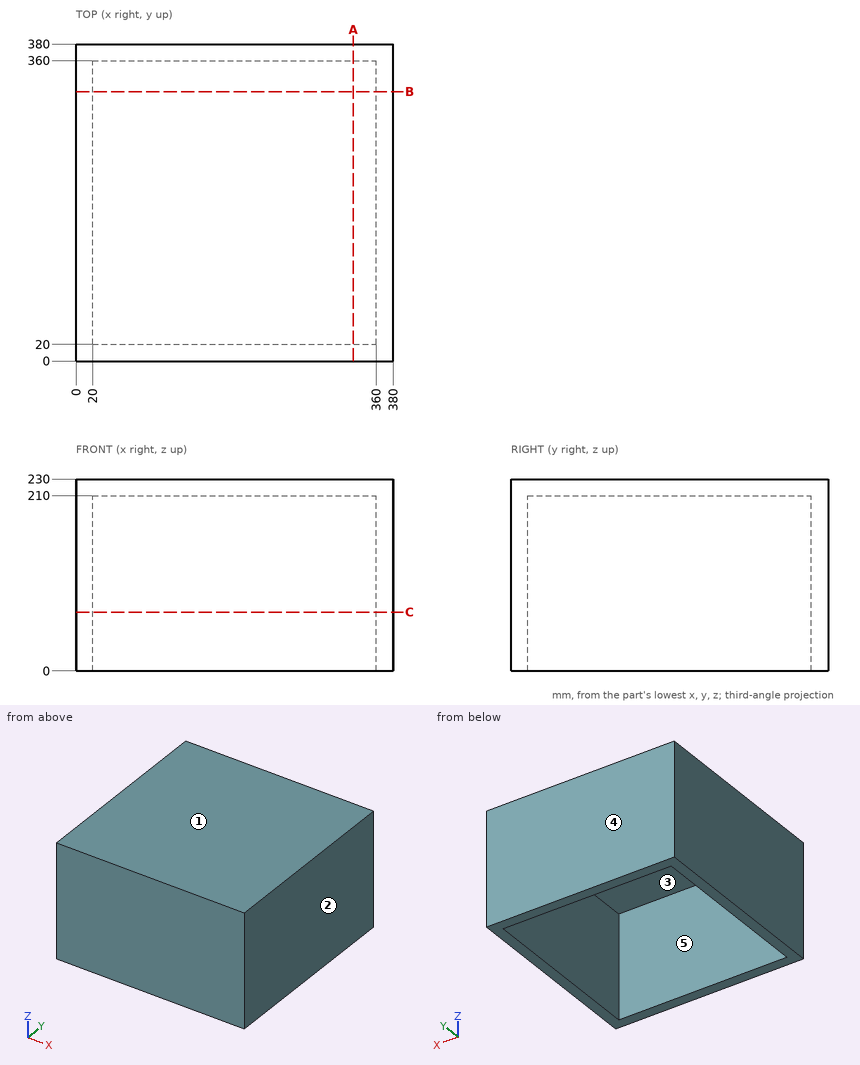
Design review of the part shown in the three views and the two pictorial views. Dimensions are in mm from the part's minimum x, y and z. A direction names the side the tool comes from. Round coordinates to 2 decimals unless told otherwise and drop trailing zeros. Loops run counter-clockwise (first coordinate to the right, second up) from the corner with the lowest first, then second, coordinate; pieces in that order, holes last. Notation, with made-up numbers: (20.5, 33) -> (71.5, 33) arc R24 ccw to (71.5, 52) -> close; hole circle Ø11 at (76.25, 49.25). An arc over 180 degrees is marked (long way). Return JSON: item names as keys, results as strings.
(1) For line 1 (X direction, y = 190, z = 71); line 2 (Z direction, x = 199.5, y = 124), list the stretches that pass through material, from the lowest coordinate up.
Solved:
{"line 1": "0 to 20, 360 to 380", "line 2": "210 to 230"}
(2) Add section A-A on x = 332.5. Write out the cut boundary in (y, z), plus the area to 3 significant figures.
Solved:
{"outline": "(0, 0) -> (20, 0) -> (20, 210) -> (360, 210) -> (360, 0) -> (380, 0) -> (380, 230) -> (0, 230) -> close", "area": "16,000 mm2"}
(3) Add section C-C on z = 70.5. Write out the cut boundary in (x, y).
Solved:
{"outline": "(0, 0) -> (380, 0) -> (380, 380) -> (0, 380) -> close; hole (20, 20) -> (360, 20) -> (360, 360) -> (20, 360) -> close"}
(4) The part is to be moulded in two halves that separate along X. For the marked faces 1, 2 and 3, say which applies: released by +X, released by -X, zero draft, split by the parting line, or undercut.
Solved:
{"face 1": "zero draft", "face 2": "released by +X", "face 3": "undercut"}
(5) For the marked faces 4 and 5, list the 3-axis set-ups (+Z, -Z, +X, -X, +Y, -Y) from which the entire face can be reached by the end or side of a thin tool; tool diameter is ignored.
Solved:
{"face 4": "+Z, -Z, +X, -X, +Y", "face 5": "-Z"}
(6) For pin 1 (4 mm diameter, centred on x = 156.5, y = 324, fed in from -Z), flat-tipped, find the tip position at first contact; note if it passes through.
Solved:
{"pin 1": "z = 210"}
